from build123d import *

# Parameters (mm, degrees)
BOSS_EXTRUDE1_DEPTH = 12.7
FILLET1_R           = 12.7
BOSS_EXTRUDE2_DEPTH = 2.54
FILLET2_R           = 6.35
SKETCH3_R           = 6.35
SKETCH3_W           = 128.842678874
SKETCH3_H           = 12.7
BOSS_EXTRUDE3_DEPTH = 2.54
FILLET3_R           = 1.5875


with BuildPart() as part:
    # Sketch1 → Boss-Extrude1 (new body)
    with BuildSketch(Plane(origin=(0, 0, 0), x_dir=(1, 0, 0), z_dir=(0, 1, 0))):
        with BuildLine():
            Line((-101.6, 0), (101.6, 0))
            ThreePointArc((101.6, 0), (96.863119244, -108.334556213), (82.688632431, -215.842221209))
            Line((82.688632431, -215.842221209), (-117.415334702, -180.506087613))
            ThreePointArc((-117.415334702, -180.506087613), (-105.561392761, -90.598803078), (-101.6, 0))
        make_face()
    extrude(amount=BOSS_EXTRUDE1_DEPTH)

    # Fillet1
    fillet1_edges = [part.edges().sort_by_distance(p)[0] for p in [
        (82.688632431, 6.35, 215.842221209),
        (-117.415334702, 6.35, 180.506087613),
    ]]
    fillet(fillet1_edges, radius=FILLET1_R)

    # Sketch2 → Boss-Extrude2 (add)
    with BuildSketch(Plane(origin=(0, 12.7, 0), x_dir=(1, 0, 0), z_dir=(0, 1, 0))):
        Polygon((-54.61463437, -178.699496428), (-23.348389506, -184.220767302), (-19.814776146, -164.210370589), (-29.819974503, -162.443563909), (-31.586781182, -172.448762265), (-42.842629334, -170.461104751), (-37.542209294, -140.445509681), (-26.286361143, -142.433167195), (-28.053167823, -152.438365552), (-18.047969466, -154.205172232), (-14.514356107, -134.194775519), (-45.780600971, -128.673504644), align=None)
        Polygon((-98.387377181, -170.969717203), (-67.121132316, -176.490988078), (-63.587518956, -156.480591364), (-73.592717313, -154.713784685), (-75.359523993, -164.718983041), (-86.615372144, -162.731325527), (-81.314952105, -132.715730457), (-70.059103953, -134.703387971), (-71.825910633, -144.708586328), (-61.820712277, -146.475393008), (-58.287098917, -126.464996294), (-89.553343782, -120.94372542), align=None)
    extrude(amount=BOSS_EXTRUDE2_DEPTH)

    # Fillet2
    fillet2_edges = [part.edges().sort_by_distance(p)[0] for p in [
        (-67.121132316, 13.97, 176.490988078),
        (-58.287098917, 13.97, 126.464996294),
        (-89.553343782, 13.97, 120.94372542),
        (-98.387377181, 13.97, 170.969717203),
        (-23.348389506, 13.97, 184.220767302),
        (-14.514356107, 13.97, 134.194775519),
        (-45.780600971, 13.97, 128.673504644),
        (-54.61463437, 13.97, 178.699496428),
    ]]
    fillet(fillet2_edges, radius=FILLET2_R)

    # Sketch3 → Boss-Extrude3 (add)
    with BuildSketch(Plane(origin=(0, 12.7, 0), x_dir=(1, 0, 0), z_dir=(0, 1, 0))):
        with Locations((-84.061485004, -74.95573952)):
            Circle(SKETCH3_R)
        with Locations((54.755611036, -102.677273515)):
            Circle(SKETCH3_R)
        with Locations((-81.443399967, -20.868490804)):
            Circle(SKETCH3_R)
        with Locations((60.495827673, -43.728490804)):
            Circle(SKETCH3_R)
        Polygon((-65.244701553, -81.966706683), (61.677933479, -86.398942765), (62.121157087, -73.706679262), (-64.801477945, -69.27444318), align=None)
        Polygon((-91.427031054, -103.926333773), (35.495603978, -108.358569854), (35.938827586, -95.666306351), (-90.983807446, -91.23407027), align=None)
        with Locations((4.18018601, -20.868490804)):
            Rectangle(SKETCH3_W, SKETCH3_H)
        with Locations((-23.37206053, -43.728490804)):
            Rectangle(SKETCH3_W, SKETCH3_H)
        Polygon((-84.153810009, 0), (-83.882599151, -4.769682556), (0, 0), align=None)
    extrude(amount=BOSS_EXTRUDE3_DEPTH)

    # Fillet3
    fillet3_edges = [part.edges().sort_by_distance(p)[0] for p in [
        (-64.801477945, 13.97, 69.27444318),
        (-65.244701553, 13.97, 81.966706683),
        (61.677933479, 13.97, 86.398942765),
        (62.121157087, 13.97, 73.706679262),
        (-83.882599151, 13.97, 4.769682556),
        (-90.983807446, 13.97, 91.23407027),
        (-91.427031054, 13.97, 103.926333773),
        (35.495603978, 13.97, 108.358569854),
        (35.938827586, 13.97, 95.666306351),
        (-60.241153427, 13.97, 14.518490804),
        (-60.241153427, 13.97, 27.218490804),
        (68.601525447, 13.97, 27.218490804),
        (68.601525447, 13.97, 14.518490804),
        (-87.793399967, 13.97, 37.378490804),
        (-87.793399967, 13.97, 50.078490804),
        (41.049278907, 13.97, 50.078490804),
        (41.049278907, 13.97, 37.378490804),
    ]]
    fillet(fillet3_edges, radius=FILLET3_R)


solid = part.part
Check sheet for the modelled part. Datum: model origin and axes. Units: mm. A direction names the side the tool comes from. Round coordinates to 2 decimals unless told otherwise and drop trailing zeros. Order: outer loops, then holes, each group sorted by start corner. A loop starts at its lowest first (then second) coordinate and runs counter-clockwise, first axis right, second up.
(1) Access from +Z, -Z, +X, -X, +Y, -Y to the whole of each face (thin tool, end or side, straight path). Record for faces 4 (the flat face through (-84, 13.95, 147.93)), 5 (the flat face through (60, 15.24, 44)), 6 (the flat face through (-41.725, 13.952, 2.373)).
(2) Cross-section at D-D, the plane x = -13. Enter the section's corners in (y, z), and give its area (3 significant figures).
(3) Cross-section at B-B, the plane x = 57. Enter the section's corners in (y, z).
(4) Scan lines: probe 1 along Y at (x, z) = (56, 166.5); probe 2 along Z at (x, y) = (-4, 14.75); probe 3 along Z at (x, y) = (59, 12.75). Record each from-to range of solid material in increasing order.
(5) Draft check along Z on faces 1 (the cylindrical face through (-85.438, 13.952, 81.155)), 2 (the cylindrical face through (-68.572, 13.988, 174.296)), 3 (the flat face through (-82, 15.24, 21)). Enter one of: pulls with the +Z half, pulls with the -Z half, needs draft (parallel to the pull), parting line crosses it, or undercut.
(6) Cross-section at A-A, the plane y = 3. Enter the section's corners in (x, z).
(7) Go/stop test with flat-tipped pins: P1, Ø2, axis at y = 14, z = 42, coming from the +X side; P2, Ø0.8, axis at y = 13.5, z = 42, coming from the -X side; P3, Ø1, axis at x = -78.5, y = 2, coming from the +Z side. Record where each tip stops, or that it passes through.
(8) Cross-section at C-C, the plane z = 197. Enter the section's corners in (x, y), and give its area (3 significant figures).
Check sheet entries:
1. face 4: +Y
1. face 5: +Z, -Z, +X, -X, +Y
1. face 6: +X, +Y
2. outline: (0, 0) - (15.24, 0) - (15.24, 0.74) - (12.7, 0.74) - (12.7, 14.52) - (15.24, 14.52) - (15.24, 27.22) - (12.7, 27.22) - (12.7, 37.38) - (15.24, 37.38) - (15.24, 50.08) - (12.7, 50.08) - (12.7, 71.08) - (15.24, 71.08) - (15.24, 83.79) - (12.7, 83.79) - (12.7, 93.96) - (15.24, 93.96) - (15.24, 106.67) - (12.7, 106.67) - (12.7, 198.94) - (0, 198.94) - close
2. area: 2,660 mm2
3. outline: (0, 0) - (12.7, 0) - (12.7, 14.52) - (15.24, 14.52) - (15.24, 27.22) - (12.7, 27.22) - (12.7, 38.43) - (15.24, 38.43) - (15.24, 49.03) - (12.7, 49.03) - (12.7, 73.53) - (15.24, 73.53) - (15.24, 86.24) - (12.7, 86.24) - (12.7, 96.74) - (15.24, 96.74) - (15.24, 108.62) - (12.7, 108.62) - (12.7, 211.31) - (0, 211.31) - close
4. probe 1: y = 0 to 12.7
4. probe 2: z = 0 to 0.23, 14.52 to 27.22, 37.38 to 50.08, 71.4 to 84.11, 94.27 to 106.98
4. probe 3: z = 14.52 to 27.22, 37.56 to 49.9, 73.6 to 86.31, 97.95 to 107.4
5. face 1: undercut
5. face 2: pulls with the +Z half
5. face 3: needs draft
6. outline: (-115.31, 168.14) arc R1038 cw to (-101.6, 0) - (101.6, 0) arc R1241.2 ccw to (84.85, 203.19) arc R12.7 ccw to (70.12, 213.62) - (-104.98, 182.7) arc R12.7 ccw to start
7. P1: stops at x = 66.8
7. P2: stops at x = -87.79
7. P3: stops at z = 187.47
8. outline: (-24.01, 0) - (85.87, 0) - (85.87, 12.7) - (-24.01, 12.7) - close
8. area: 1,400 mm2
